Work out the finished part from the listing and answer in its coordinate system (mm). Give positions to 0.01 mm unless a question says otherwise; leave off trailing zeros. Write each loop counter-clockwise with the first axis right and the second up, starting at its lowest first coordinate (ties: lowest second). Pieces come first, ordered by that corner, then holes. Notation, with made-up numbers: (-37.75, 27) -> (-13.75, 27) arc R28 cw to (-13.75, 59) -> close; hole circle Ø9 at (64.5, -12.75). An arc over 180 degrees is marked (long way). Use a Markdown table: item, result. Add a question column.
Q1. Each of these flat-tipped pins is pushed along its axis until it touches: pin 1 Ø10 at (x, z) = (146, -63) entering from -Y; pin 2 Ø1 at (x, y) = (708, 14.5) entering from +Z. Where does it stop, or does it pass through?
Q2. Section B-B, the plane y = 8.75 is taken. Give the vertices of the cut face in (x, z).
Q3. Section C-C, the plane x = 217 is taken. Give the vertices of the cut face in (y, z), plus the area to 3 significant figures.
Q4. Section A-A, the plane z = -84 is taken. Give the vertices of the cut face in (x, y).
Q5. For a pull along Z with two mould halves and no side action, classify faces 1 (the face through (714.49, 9.66, -86.41)), 2 (the face through (369, 19.05, -68)), 3 (the face through (603.155, 9.658, -86.299)), 4 (the face through (369, 9, -149.282)) as pulls with the +Z half, pulls with the -Z half, needs draft (parallel to the pull), parting line crosses it, or undercut.
Q6. Consider line 1 (X direction, y = 15.25, z = -83); line 2 (X direction, y = 9.5, z = -99.5); line 3 (Z direction, x = 319, y = 17.5). Determine where each line is inside the solid, lowest interval first.
from build123d import *

# Parameters (mm, degrees)
SKETCH1_W           = 876.3
SKETCH1_H           = 165.1
BOSS_EXTRUDE1_DEPTH = 19.05
SKETCH3_R           = 29.499999928
CUT_EXTRUDE1_DEPTH  = 19.05
SKETCH2_R           = 29.499999928
CUT_EXTRUDE2_DEPTH  = 19.05
CUT_EXTRUDE3_DEPTH  = 914.4


with BuildPart() as part:
    # Sketch1 → Boss-Extrude1 (new body)
    with BuildSketch(Plane(origin=(0, 0, 0), x_dir=(1, 0, 0), z_dir=(0, 1, 0))):
        with Locations((375.34945696, 66.731818106)):
            Rectangle(SKETCH1_W, SKETCH1_H)
    extrude(amount=BOSS_EXTRUDE1_DEPTH)

    # Sketch3 → Cut-Extrude1 (cut)
    with BuildSketch(Plane(origin=(0, 19.05, 0), x_dir=(1, 0, 0), z_dir=(0, 1, 0))):
        with Locations(Location((573.905935058, 82.4588113, 0), (0, 0, 270))):
            Circle(SKETCH3_R)
    extrude(amount=-CUT_EXTRUDE1_DEPTH, mode=Mode.SUBTRACT)

    # Sketch2 → Cut-Extrude2 (cut)
    with BuildSketch(Plane(origin=(0, 19.05, 0), x_dir=(1, 0, 0), z_dir=(0, 1, 0))):
        with Locations(Location((685.24027425, 82.567946762, 0), (0, 0, 270))):
            Circle(SKETCH2_R)
    extrude(amount=-CUT_EXTRUDE2_DEPTH, mode=Mode.SUBTRACT)

    # Sketch4 → Cut-Extrude3 (cut)
    with BuildSketch(Plane.ZY.offset(62.80054304)):
        Polygon((-3.231818106, 0), (15.818181894, 19.05), (15.818181894, 0), align=None)
    extrude(amount=-CUT_EXTRUDE3_DEPTH, mode=Mode.SUBTRACT)


solid = part.part
Result set:
| question | item | result |
|---|---|---|
| 1 | pin 1 | stops at y = 0 |
| 1 | pin 2 | stops at z = 11.77 |
| 2 | outline | (-62.8, -149.28) -> (813.5, -149.28) -> (813.5, 5.52) -> (-62.8, 5.52) -> close; hole circle Ø59 at (573.91, -82.46); hole circle Ø59 at (685.24, -82.57) |
| 3 | outline | (0, -149.28) -> (19.05, -149.28) -> (19.05, 15.82) -> (0, -3.23) -> close |
| 3 | area | 2,960 mm2 |
| 4 | outline | (-62.8, 0) -> (544.45, 0) -> (544.45, 19.05) -> (-62.8, 19.05) -> close; (603.37, 0) -> (655.78, 0) -> (655.78, 19.05) -> (603.37, 19.05) -> close; (714.71, 0) -> (813.5, 0) -> (813.5, 19.05) -> (714.71, 19.05) -> close |
| 5 | face 1 | undercut |
| 5 | face 2 | needs draft |
| 5 | face 3 | undercut |
| 5 | face 4 | pulls with the -Z half |
| 6 | line 1 | x = -62.8 to 544.41, 603.4 to 655.74, 714.74 to 813.5 |
| 6 | line 2 | x = -62.8 to 549.83, 597.99 to 661.08, 709.4 to 813.5 |
| 6 | line 3 | z = -149.28 to 14.27 |
